```python
from build123d import *

# Parameters (mm, degrees)
F0_W     = 30
F0_H     = 75
F1_DEPTH = 2.5
F2_R     = 4.99999


# Not quite as in the source:
# - a fillet or chamfer is up to 0.001 mm smaller than in the source, because OpenCascade refuses the exact size


with BuildPart() as f1:
    # F0 (on Top) → F1 (new body, symmetric)
    with BuildSketch(Plane.XY):
        Rectangle(F0_W, F0_H)
    extrude(amount=F1_DEPTH, both=True)

    # F2 (radius 5 in the source; OpenCascade refuses exactly that, so slightly less here)
    f2_edges = [f1.edges().sort_by_distance(p)[0] for p in [
        (15, 0, 2.5),
        (-15, 0, 2.5),
    ]]
    fillet(f2_edges, radius=F2_R)


solid = f1.part
```
Input: part model. Units: mm. Frame: model coordinates. Round coordinates to 2 decimals unless told otherwise and drop trailing zeros. Loops run counter-clockwise (first coordinate to the right, second up) from the corner with the lowest first, then second, coordinate; pieces in that order, holes last. Notation, with made-up numbers: (59.5, -18) -> (64.5, -18) arc R20 cw to (64.5, 21) -> close; hole circle Ø6 at (54, -35.5). An arc over 180 degrees is marked (long way). One line per item, written item: value.
(1) Material intervals for line 1 (X direction, y = 6, z = 0.1); line 2 (X direction, y = -3, z = 1.4); line 3 (Z direction, x = 13.75, y = -29), sorted ascending. Write a range as [from, to].
Geometry check:
line 1: [-14.27, 14.27]
line 2: [-13.13, 13.13]
line 3: [-2.5, 0.81]
(2) Section C-C (x = -12). Return the cut outline in (y, z).
Geometry check:
outline: (-37.5, -2.5) -> (37.5, -2.5) -> (37.5, 2.08) -> (-37.5, 2.08) -> close
(3) Section B-B (z = 1.5). Return the cut outline in (x, y), plus the area to 3 significant figures.
Geometry check:
outline: (-13, -37.5) -> (13, -37.5) -> (13, 37.5) -> (-13, 37.5) -> close
area: 1,950 mm2
